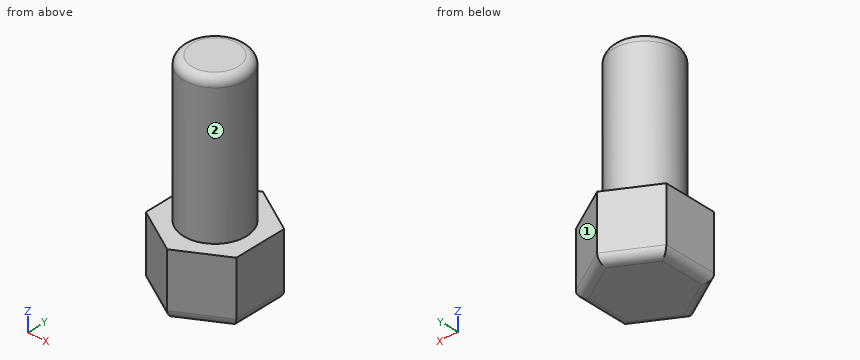
```python
from build123d import *

# Parameters (mm, degrees)
F1_DEPTH = 3
F2_R     = 1.5
F3_DEPTH = 7
F4_R     = 0.4


with BuildPart() as f1:
    # F0 (on Top) → F1 (new body)
    with BuildSketch(Plane.XY):
        Polygon((2.165064, 1.25), (0, 2.5), (-2.165064, 1.25), (-2.165064, -1.25), (0, -2.5), (2.165064, -1.25), align=None)
    extrude(amount=F1_DEPTH)

    # F2 (on face) → F3 (join)
    with BuildSketch(Plane.XY.offset(3)):
        Circle(F2_R)
    extrude(amount=F3_DEPTH)

    # F4
    f4_edges = [f1.edges().sort_by_distance(p)[0] for p in [
        (-1.082532, 1.875, 0),
        (-2.165064, 0, 0),
        (-1.082532, -1.875, 0),
        (1.082532, -1.875, 0),
        (2.165064, 0, 0),
        (1.082532, 1.875, 0),
        (-1.5, 0, 10),
    ]]
    fillet(f4_edges, radius=F4_R)


solid = f1.part
```
Here's how the part is built. I have some questions about the finished solid (model axes, mm). Face numbers are marked on the shaded views. A direction names the side the tool comes from. Coordinates: 2 decimals unless noted, no trailing zeros. Loops run counter-clockwise (first coordinate to the right, second up) from the corner with the lowest first, then second, coordinate; pieces in that order, holes last. Notation, with made-up numbers: (-9, 82.25) - (-2, 82.25) arc R35 cw to (-2, 119.25) - close; hole circle Ø6 at (-12, 24). An arc over 180 degrees is marked (long way). Return JSON: item names as keys, results as strings. Group by question number.
Item 1: Will these pins go through, and if not, where does the flat tip stop? P1, Ø2, axis at y = 2, z = 8, coming from the -X side; P2, Ø1, axis at y = 1.5, z = 4.5, coming from the +X side.
Item 2: If we section it at B-B on z = 1: Write out the boundary of the cut face in (x, y), and give its area (3 significant figures).
Item 3: On a 3-axis mill with a long thin cutter (end or side, diameter ignored), from which of +Z, -Z, +X, -X, +Y, -Y can I reach the whole of each face in a straight line? I mean the marked faces 1 and 2. Say none if no direction works.
Item 4: I need wall thicknesses on line 1 (Z direction, x = 1.2, y = -1.25); line 2 (Y direction, x = 1.2, z = 9.5); line 3 (Y direction, x = -1.05, z = 5). Which ranges of each line are inside material? Lowest first, please. Write a range as from..to.
Item 5: If we section it at A-A on y = 0: Write out the boundary of the cut face in (x, z), and give its area (3 significant figures).
Item 6: If we section it at C-C on z = 6.75: Write out the boundary of the cut face in (x, y).
Calculated:
{
 "1": {"P1": "stops at x = -1.12", "P2": "stops at x = 1.12"},
 "2": {"outline": "(-2.17, -1.25) - (0, -2.5) - (2.17, -1.25) - (2.17, 1.25) - (0, 2.5) - (-2.17, 1.25) - close", "area": "16.2 mm^2"},
 "3": {"face 1": "+Z, -Z, +X, +Y", "face 2": "+Z"},
 "4": {"line 1": "z = 0..3", "line 2": "y = -0.9..0.9", "line 3": "y = -1.07..1.07"},
 "5": {"outline": "(-2.17, 0.4) arc R0.4 ccw to (-1.77, 0) - (1.77, 0) arc R0.4 ccw to (2.17, 0.4) - (2.17, 3) - (1.5, 3) - (1.5, 9.6) arc R0.4 ccw to (1.1, 10) - (-1.1, 10) arc R0.4 ccw to (-1.5, 9.6) - (-1.5, 3) - (-2.17, 3) - close", "area": "33.9 mm^2"},
 "6": {"outline": "circle Ø3 at (0, 0)"}
}
